Autodesk Inventor part; units mm, degrees
ref_plane "YZ Plane" through (0, 0, 0) normal (1, 0, 0) x (0, 1, 0)
ref_plane "XZ Plane" through (0, 0, 0) normal (0, 1, 0) x (-1, 0, 0)
ref_plane "XY Plane" through (0, 0, 0) normal (0, 0, 1) x (1, 0, 0)
sketch "Sketch1" plane through (0, 0, 0) normal (0, 0, 1) x (1, 0, 0)
  line L0 (222.25, 25.4) -> (-222.25, 25.4)
  line L1 (-222.25, 25.4) -> (-222.25, -25.4)
  line L2 (-222.25, -25.4) -> (222.25, -25.4)
  line L3 (222.25, -25.4) -> (222.25, 25.4)
  line L4 (222.25, 25.4) -> (-222.25, -25.4) construction
  line L5 (-222.25, 25.4) -> (222.25, -25.4) construction
  point P0 (0, 0)
  dimension "d0" = 444.5
  dimension "d1" = 50.8
extrude "Extrusion1" add sketch "Sketch1" along normal blind 25.4
sketch "Sketch2" plane through (0, 0, 25.4) normal (0, 0, 1) x (1, 0, 0)
  point P0 (0, -3.175)
  point P1 (0, -3.175)
  point P2 (-190.5, 0)
  point P3 (190.5, 0)
  point P4 (0, 0)
  dimension "d4" = 3.175
  dimension "d5" = 190.5
  dimension "d6" = 190.5
  dimension "d7" = 3.175
shell "Shell1" thickness 2.54 removed faces 2 at (222.25, -8.4667, 8.4667) at (-222.25, 8.4667, 16.9333)
hole "Hole1" at (0, -3.175, 25.4) at (-190.5, 0, 25.4) at (190.5, 0, 25.4) direction (0, 0, -1) diameter 8.1026 end through all
properties part number "Drive base"
Geometry: final body of the model. Coordinates: model frame, mm. A direction names the side the tool comes from. Coordinates: 2 decimals unless noted, no trailing zeros. Order: outer loops, then holes, each group sorted by start corner. A loop starts at its lowest first (then second) coordinate and runs counter-clockwise, first axis right, second up. Notation, with made-up numbers: (67.25, 78.25) - (82.25, 78.25) arc R4 ccw to (82.25, 85.25) - close; hole circle Ø2 at (7.5, -1.5). An arc over 180 degrees is marked (long way). Return JSON: item names as keys, results as strings. Group by question number.
1. Pull-direction query (Y, two-part tool) for faces 1 (the face through (-3, 0, 22.86)), 2 (the face through (-3, -25.4, 13)), 3 (the face through (222.25, 0, 2)); classes: pulls with the +Y half, pulls with the -Y half, needs draft (parallel to the pull), parting line crosses it, or undercut.
2. Material intervals for line 1 along Z through (x, y) = (-41, -6); line 2 along Y through (x, z) = (0, 0.5); line 3 along Y through (x, z) = (37.5, 7), sorted ascending. Write a range as [from, to].
3. Cut plane C-C (y = -15). Output: boundary loops of the cut face in (x, z), plus the area to 3 significant figures.
4. Cut plane D-D (x = -178). Output: boundary loops of the cut face in (y, z).
5. Cut plane B-B (x = 190.5). Output: boundary loops of the cut face in (y, z).
6. Pin query (flat end, axial travel): pin 1 (4 mm diameter, centred on y = -19.5, z = 8.5, fed in from +X). Return the tip coordinate at first contact, or that it passes through.
7. Cut plane A-A (z = 18). Output: boundary loops of the cut face in (x, y).
8. Set-up query: faces 4 (the face through (-194.517, 0.527, 24.112)), 5 (the face through (-3, -22.86, 13)). Return all of +Z, -Z, +X, -X, +Y, -Y with unobstructed straight access to the full face (end or side cutting, diameter ignored); none if empty.
Resolved:
{
 "1": {"face 1": "undercut", "face 2": "pulls with the -Y half", "face 3": "needs draft"},
 "2": {"line 1": "z = [0, 2.54], [22.86, 25.4]", "line 2": "y = [-25.4, -7.23], [0.88, 25.4]", "line 3": "y = [-25.4, -22.86], [22.86, 25.4]"},
 "3": {"outline": "(-222.25, 0) - (222.25, 0) - (222.25, 2.54) - (-222.25, 2.54) - close; (-222.25, 22.86) - (222.25, 22.86) - (222.25, 25.4) - (-222.25, 25.4) - close", "area": "2,260 mm²"},
 "4": {"outline": "(-25.4, 0) - (25.4, 0) - (25.4, 25.4) - (-25.4, 25.4) - close; hole (-22.86, 2.54) - (22.86, 2.54) - (22.86, 22.86) - (-22.86, 22.86) - close"},
 "5": {"outline": "(-25.4, 0) - (-4.05, 0) - (-4.05, 2.54) - (-22.86, 2.54) - (-22.86, 22.86) - (-4.05, 22.86) - (-4.05, 25.4) - (-25.4, 25.4) - close; (4.05, 0) - (25.4, 0) - (25.4, 25.4) - (4.05, 25.4) - (4.05, 22.86) - (22.86, 22.86) - (22.86, 2.54) - (4.05, 2.54) - close"},
 "6": {"pin 1": "passes through"},
 "7": {"outline": "(-222.25, -25.4) - (222.25, -25.4) - (222.25, -22.86) - (-222.25, -22.86) - close; (-222.25, 22.86) - (222.25, 22.86) - (222.25, 25.4) - (-222.25, 25.4) - close"},
 "8": {"face 4": "+Z, -Z", "face 5": "+X, -X"}
}
